Here's how the part is built. I have some questions about the finished solid (model axes, mm). Face numbers are marked on the shaded views. A direction names the side the tool comes from. Round coordinates to 2 decimals unless told otherwise and drop trailing zeros. Loops run counter-clockwise (first coordinate to the right, second up) from the corner with the lowest first, then second, coordinate; pieces in that order, holes last. Notation, with made-up numbers: (67, 25) -> (87, 25) arc R33 cw to (87, 61) -> close; hole circle Ø8 at (86.5, -28.75). An arc over 180 degrees is marked (long way). Use CSV: the item, a comma, the result in double quotes. Start each with the question number.
from build123d import *

# Parameters (mm, degrees)
F0_R     = 37.250135
F1_DEPTH = 50.8
F2_W     = 11.076774
F2_H     = 12.752968
F2_W_2   = 17.722838
F2_H_2   = 15.002562
F3_DEPTH = 50.8
F4_W     = 13.871703
F4_H     = 15.605667


with BuildPart() as f1:
    # F0 (on Front) → F1 (new body)
    with BuildSketch(Plane.XZ):
        Circle(F0_R)
    extrude(amount=F1_DEPTH)

    # F2 (on face) → F3 (cut)
    with BuildSketch(Plane.XZ.offset(50.8)):
        with Locations((-17.74689, 11.526265)):
            Rectangle(F2_W, F2_H)
        with Locations((13.489608, -7.501281)):
            Rectangle(F2_W_2, F2_H_2)
    extrude(amount=-F3_DEPTH, mode=Mode.SUBTRACT)

    # F4 (on Top) → F6 (revolve, cut)
    with BuildSketch(Plane.XY):
        with Locations((-35.360457, -14.181339)):
            Rectangle(F4_W, F4_H)
    revolve(axis=Axis((0, 18.854436, 0), (0, 1, 0)), mode=Mode.SUBTRACT)


solid = f1.part
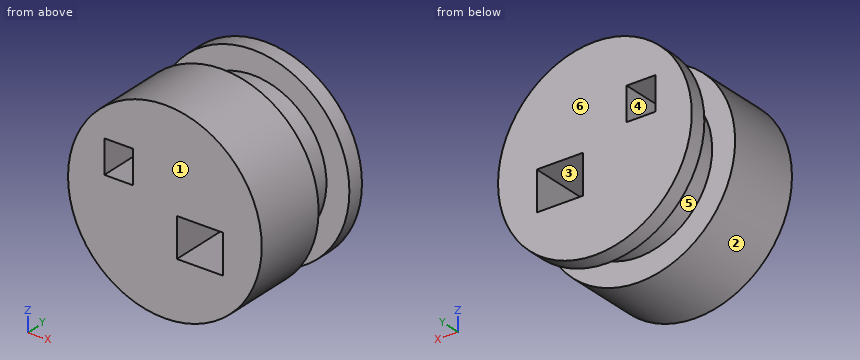
Q1. I want a section at B-B, the plane y = -26. List the corners of the cut face in (x, z) for me, then the cut area to 3 significant figures.
Q2. I want a section at C-C, the plane z = -9. List the corners of the cut face in (x, y) for me.
Q3. I need wall thicknesses on line 1 along Y through (x, z) = (15.5, 28); line 2 along Z through (x, y) = (-19.5, -29); line 3 along X through (y, z) = (-10.5, -8). Which ranges of each line are inside material? Lowest first, please.
Q4. I want a section at A-A, the plane x = 0. List the corners of the cut face in (y, z) for me, then the cut area to 3 significant figures.
Q5. For the marked faces 4, 5 and 6, which set-ups out of +Z, -Z, +X, -X, +Y, -Y let a thin tool reach every point of the face, with its end or its side?
Q6. I want a section at D-D, the plane x = -17.5. List the corners of the cut face in (y, z) for me, then the cut area to 3 significant figures.
Q7. If we mould it in two halves opening along Z, with no side actions, what happens to the marked faces 1, 2 and 3? For each: pulls with the +Z half, pulls with the -Z half, needs draft (parallel to the pull), parting line crosses it, or undercut.
Q8. Will these pins go through, and if not, where does the flat tip stop? pin 1 Ø2 at (x, y) = (-7.5, -38) entering from +Z; pin 2 Ø10 at (y, z) = (-22.5, 10) entering from +X; pin 3 Ø4 at (y, z) = (-28, 22.5) entering from -X.
Values found:
1,outline,"circle Ø74.5 at (0, 0); hole (-23.29, 5.15) -> (-12.21, 5.15) -> (-12.21, 17.9) -> (-23.29, 17.9) -> close; hole (4.63, -15) -> (22.35, -15) -> (22.35, 0) -> (4.63, 0) -> close"
1,area,"3,950 mm2"
2,outline,"(-36.15, -50.8) -> (4.63, -50.8) -> (4.63, 0) -> (-36.15, 0) -> (-36.15, -6.38) -> (-26.96, -6.38) -> (-26.96, -21.98) -> (-36.15, -21.98) -> close; (22.35, -50.8) -> (36.15, -50.8) -> (36.15, -21.98) -> (26.96, -21.98) -> (26.96, -6.38) -> (36.15, -6.38) -> (36.15, 0) -> (22.35, 0) -> close"
3,line 1,"-50.8 to -21.98, -6.38 to 0"
3,line 2,"-31.74 to 5.15, 17.9 to 31.74"
3,line 3,"-27.28 to 4.63, 22.35 to 27.28"
4,outline,"(-50.8, -37.25) -> (-21.98, -37.25) -> (-21.98, -28.42) -> (-6.38, -28.42) -> (-6.38, -37.25) -> (0, -37.25) -> (0, 37.25) -> (-6.38, 37.25) -> (-6.38, 28.42) -> (-21.98, 28.42) -> (-21.98, 37.25) -> (-50.8, 37.25) -> close"
4,area,"3,510 mm2"
5,face 4,"+Y, -Y"
5,face 5,"none"
5,face 6,"+Z, -Z, +X, -X, +Y"
6,outline,"(-50.8, -32.88) -> (-21.98, -32.88) -> (-21.98, -22.4) -> (-6.38, -22.4) -> (-6.38, -32.88) -> (0, -32.88) -> (0, 5.15) -> (-50.8, 5.15) -> close; (-50.8, 17.9) -> (0, 17.9) -> (0, 32.88) -> (-6.38, 32.88) -> (-6.38, 22.4) -> (-21.98, 22.4) -> (-21.98, 32.88) -> (-50.8, 32.88) -> close"
6,area,"2,370 mm2"
7,face 1,"needs draft"
7,face 2,"parting line crosses it"
7,face 3,"undercut"
8,pin 1,"z = 36.68"
8,pin 2,"x = 36.91"
8,pin 3,"x = -31.1"
